Work out the finished part from the listing and answer in its coordinate system (mm). A direction names the side the tool comes from. Give positions to 0.01 mm unless a question says otherwise; leave off trailing zeros. Loops run counter-clockwise (first coordinate to the right, second up) from the corner with the lowest first, then second, coordinate; pieces in that order, holes last.
```python
from build123d import *

# Parameters (mm, degrees)
SKETCH2_W           = 12.7
SKETCH2_H           = 25.4
BOSS_EXTRUDE2_DEPTH = 57.15
SKETCH3_W           = 10.16
SKETCH3_H           = 76.2
BOSS_EXTRUDE3_DEPTH = 25.4


with BuildPart() as part:
    # Sketch2 → Boss-Extrude2 (new body)
    with BuildSketch(Plane(origin=(0, 0, 0), x_dir=(1, 0, 0), z_dir=(0, 1, 0))):
        with Locations((0, -12.7)):
            Rectangle(SKETCH2_W, SKETCH2_H)
    extrude(amount=BOSS_EXTRUDE2_DEPTH)



with BuildPart() as body_2:
    # Sketch3 → Boss-Extrude3 (new body)
    with BuildSketch(Plane(origin=(0, 0, 0), x_dir=(1, 0, 0), z_dir=(0, 1, 0))):
        with Locations((0, -368.3)):
            Rectangle(SKETCH3_W, SKETCH3_H)
    extrude(amount=BOSS_EXTRUDE3_DEPTH)


with BuildPart() as part_1:
    add(part.part)

    add(body_2.part)  # Revolve2 merges body 2
    # Sketch4 → Revolve2 (revolve)
    with BuildSketch(Plane(origin=(0, 0, 0), x_dir=(0, 0, -1), z_dir=(1, 0, 0)), mode=Mode.PRIVATE) as revolve2_sk:
        with BuildLine():
            Line((0, 0), (0, 50.8))
            Line((0, 50.8), (-25.4, 50.8))
            Line((-25.4, 50.8), (-25.4, 31.75))
            ThreePointArc((-25.4, 31.75), (-29.119743879, 22.769743879), (-38.1, 19.05))
            Line((-38.1, 19.05), (-406.4, 19.05))
            Line((-406.4, 19.05), (-406.4, 0))
            Line((-406.4, 0), (0, 0))
        make_face()
    revolve(revolve2_sk.sketch.rotate(Axis((0, 0, 1000), (0, 0, -1)), 90), axis=Axis((0, 0, 1000), (0, 0, -1)))


solid = part_1.part
```
Q1. Section C-C on z = 194.5 is taken. Give the vertices of the cut face in (x, y).
Q2. Section D-D on y = 46.5 is taken. Give the vertices of the cut face in (x, z), plus the area to 3 significant figures.
Q3. Consider line 1 along Z through (x, y) = (-35.5, 29); line 2 along Y through (x, z) = (2, 265.5); line 3 along Y through (x, z) = (-7.5, 21.5). Determine where each line is inside the solid, lowest interval first.
Q4. Which of the six approach directions +Z, -Z, +X, -X, +Y, -Y give full straight-line access (tool end or side, diameter ignored) to faces 1 (the face through (-6.35, 54, 13)), 2 (the face through (6.35, 54, 13)), 3 (the face through (0, 25.4, 368)), 4 (the face through (-5.08, 22, 369))?
Q5. Given pin 1 (3.5 mm diameter, centred on y = 54, z = 10, fed in from +X); pin 2 (3.5 mm diameter, centred on y = 23, z = 384, fed in from -X); pin 3 (6 mm diameter, centred on y = -18, z = 132, fed in from +X); pin 4 (12 mm diameter, centred on x = -25.5, z = 244.5, fed in from -Y), each flat-ended and moving along its own axis, determine where each tip first touches the part or whether it passes through.
Q6. Section B-B on y = 0 is taken. Give the vertices of the cut face in (x, z), plus the area to 3 significant figures.
Q7. Section A-A on x = 0 is taken. Give the vertices of the cut face in (y, z).
Q8. Determine the mould class of faces 5 (the face through (0, 57.15, 13)), 6 (the face through (0, 3, 406.4)), 7 (the face through (0, 22, 330.2)) for opening direction Z: +Z half, -Z half, draft (parallel to the pull), parting line (faces both ways), or undercut.
Check result:
1. outline: circle Ø38.1 at (0, 0)
2. outline: (-20.45, 0) - (20.45, 0) - (20.45, 25.4) - (-20.45, 25.4) - close
2. area: 1,040 mm2
3. line 1: z = 0 to 25.4
3. line 2: y = -18.94 to 18.94
3. line 3: y = -50.24 to 50.24
4. face 1: +Z, -Z, -X, +Y
4. face 2: +Z, -Z, +X, +Y
4. face 3: +Z, +X, -X, +Y
4. face 4: +Z, -X, +Y
5. pin 1: stops at x = 6.35
5. pin 2: stops at x = -5.08
5. pin 3: stops at x = 11.74
5. pin 4: passes through
6. outline: (-50.8, 0) - (50.8, 0) - (50.8, 25.4) - (31.75, 25.4) arc R12.7 cw to (19.05, 38.1) - (19.05, 406.4) - (-19.05, 406.4) - (-19.05, 38.1) arc R12.7 cw to (-31.75, 25.4) - (-50.8, 25.4) - close
6. area: 17,200 mm2
7. outline: (-50.8, 0) - (57.15, 0) - (57.15, 25.4) - (31.75, 25.4) arc R12.7 cw to (19.05, 38.1) - (19.05, 330.2) - (25.4, 330.2) - (25.4, 406.4) - (-19.05, 406.4) - (-19.05, 38.1) arc R12.7 cw to (-31.75, 25.4) - (-50.8, 25.4) - close
8. face 5: draft
8. face 6: +Z half
8. face 7: undercut
